Build history of the part. All positions in model axes, mm. A direction names the side the tool comes from. Give positions to 0.01 mm unless a question says otherwise; leave off trailing zeros. Order: outer loops, then holes, each group sorted by start corner. A loop starts at its lowest first (then second) coordinate and runs counter-clockwise, first axis right, second up. Notation, with made-up numbers: (73.25, 7.25) - (95.25, 7.25) arc R32 ccw to (95.25, 36.25) - close; hole circle Ø8 at (60, 25). An arc over 180 degrees is marked (long way). One line per item, written item: value.
```python
from build123d import *

# Parameters (mm, degrees)
SKETCH1_W           = 51
SKETCH1_H           = 50
BOSS_EXTRUDE1_DEPTH = 3
SKETCH2_W           = 51
SKETCH2_H           = 3
BOSS_EXTRUDE2_DEPTH = 51
SKETCH3_R           = 11
SKETCH3_R_2         = 1.5
CUT_EXTRUDE1_DEPTH  = 4
BOSS_EXTRUDE3_DEPTH = 3
CHAMFER1_SIZE       = 5


with BuildPart() as part:
    # Sketch1 → Boss-Extrude1 (new body)
    with BuildSketch(Plane(origin=(0, 0, 0), x_dir=(1, 0, 0), z_dir=(0, 1, 0))):
        Rectangle(SKETCH1_W, SKETCH1_H)
        with BuildLine():
            Line((-12.865, 15.85), (-12.865, -13.85))
            ThreePointArc((-12.865, -13.85), (-15.015, -16), (-17.165, -13.85))
            Line((-17.165, -13.85), (-17.165, 15.85))
            ThreePointArc((-17.165, 15.85), (-15.015, 18), (-12.865, 15.85))
        make_face(mode=Mode.SUBTRACT)
        with BuildLine():
            Line((12.865, 15.85), (12.865, -13.85))
            ThreePointArc((12.865, -13.85), (15.015, -16), (17.165, -13.85))
            Line((17.165, -13.85), (17.165, 15.85))
            ThreePointArc((17.165, 15.85), (15.015, 18), (12.865, 15.85))
        make_face(mode=Mode.SUBTRACT)
    extrude(amount=BOSS_EXTRUDE1_DEPTH)

    # Sketch2 → Boss-Extrude2 (add)
    with BuildSketch(Plane.XZ):
        with Locations((0, -23.5)):
            Rectangle(SKETCH2_W, SKETCH2_H)
    extrude(amount=-BOSS_EXTRUDE2_DEPTH)

    # Sketch3 → Cut-Extrude1 (cut, through all)
    with BuildSketch(Plane.XY.offset(-22)):
        with Locations((0, 30)):
            Circle(SKETCH3_R)
        with Locations((-15.5, 45.5)):
            Circle(SKETCH3_R_2)
        with Locations((15.5, 45.5)):
            Circle(SKETCH3_R_2)
        with Locations((-15.5, 14.5)):
            Circle(SKETCH3_R_2)
        with Locations((15.5, 14.5)):
            Circle(SKETCH3_R_2)
    extrude(amount=-CUT_EXTRUDE1_DEPTH, mode=Mode.SUBTRACT)

    # Sketch5 → Boss-Extrude3 (add)
    with BuildSketch(Plane.ZY.offset(25.5)):
        Polygon((-22, 23), (-2, 3), (-22, 3), align=None)
    boss_extrude3 = extrude(amount=-BOSS_EXTRUDE3_DEPTH)

    # Mirror1: Boss-Extrude3 across plane
    add(boss_extrude3.mirror(Plane(origin=(0, 0, 0), x_dir=(0, 0, 1), z_dir=(1, 0, 0))))

    # Chamfer1
    chamfer1_edges = [part.edges().sort_by_distance(p)[0] for p in [
        (-25.5, 51, -23.5),
        (25.5, 51, -23.5),
        (25.5, 1.5, 25),
        (-25.5, 1.5, 25),
    ]]
    chamfer(chamfer1_edges, length=CHAMFER1_SIZE)


solid = part.part
```
(1) 3-axis set-ups, long thin cutter, end or side, ignore diameter. For faces 4 (the face through (-15, 1, -18)), 5 (the face through (-22.5, 9, -16)), 6 (the face through (0, 0, 0)): which of +Z, -Z, +X, -X, +Y, -Y reach the whole face in a straight line?
Completed:
face 4: +Y, -Y
face 5: +Z, +Y
face 6: +Z, -Z, +X, -X, -Y
(2) Pin check, flat tips, straight feed: P1, Ø3, axis at x = -16, y = 24.5, coming from the +Z side; P2, Ø16, axis at y = 17.5, z = -11.5, coming from the +X side; P3, Ø2.5, axis at x = -15.5, y = 45.5, coming from the +Z side; P4, Ø14, axis at x = 2.5, z = -2.5, coming from the +Y side. Stop position of each tip, or through.
Completed:
P1: z = -22
P2: x = 25.5
P3: through
P4: y = 3
(3) Pull direction X, two halves, no side cores. Call faces 1 (the face through (-17, 14.57, -23.48)), 2 (the face through (-6, 19, -25)), 3 (the face through (23, 1.5, 22.5)): +X half, -X half, draft (parallel to the pull), parting line (faces both ways), or undercut.
Completed:
face 1: undercut
face 2: draft
face 3: +X half
(4) Slice it at D-D, the plane y = 30. Give the cut face in (x, z), and give its area (3 significant figures).
Completed:
outline: (-25.5, -25) - (-11, -25) - (-11, -22) - (-25.5, -22) - close; (11, -25) - (25.5, -25) - (25.5, -22) - (11, -22) - close
area: 87.0 mm²
(5) Drill centre lines: line 1 (Y direction, x = -15.5, z = -23.3); line 2 (Y direction, x = -15, z = -24); line 3 (Y direction, x = 0, z = -24.15). Where is each one in solid material? Low to high.
Completed:
line 1: 0 to 13, 16 to 44, 47 to 51
line 2: 0 to 13.09, 15.91 to 44.09, 46.91 to 51
line 3: 0 to 19, 41 to 51
(6) Slice it at C-C, the plane y = 14.5. Give the cut face in (x, z).
Completed:
outline: (-25.5, -25) - (-17, -25) - (-17, -22) - (-22.5, -22) - (-22.5, -13.5) - (-25.5, -13.5) - close; (-14, -25) - (14, -25) - (14, -22) - (-14, -22) - close; (17, -25) - (25.5, -25) - (25.5, -13.5) - (22.5, -13.5) - (22.5, -22) - (17, -22) - close
(7) Slice it at A-A, the plane x = 0. Give the cut face in (y, z), and give its area (3 significant figures).
Completed:
outline: (0, -25) - (19, -25) - (19, -22) - (3, -22) - (3, 25) - (0, 25) - close; (41, -25) - (51, -25) - (51, -22) - (41, -22) - close
area: 228 mm²
(8) Slice it at B-B, the plane z = -6.5. Give the cut face in (x, y) (3 decimals), and give its area (3 significant figures).
Completed:
outline: (-25.5, 0) - (-17.165, 0) - (-17.165, 3) - (-22.5, 3) - (-22.5, 7.5) - (-25.5, 7.5) - close; (-12.865, 0) - (12.865, 0) - (12.865, 3) - (-12.865, 3) - close; (17.165, 0) - (25.5, 0) - (25.5, 7.5) - (22.5, 7.5) - (22.5, 3) - (17.165, 3) - close
area: 154 mm²
